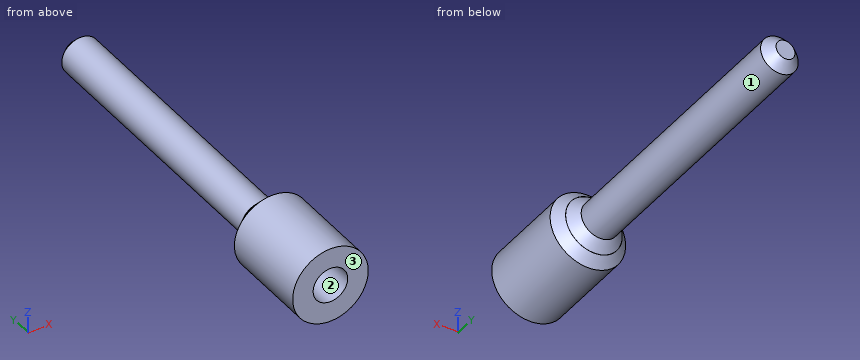
```python
from build123d import *

# Parameters (mm, degrees)
F0_R     = 101.843803
F0_R_2   = 46.640997
F1_DEPTH = 269.139469
F2_R     = 50.778729
F3_DEPTH = 801.080585
F4_SIZE  = 25.4


with BuildPart() as f1:
    # F0 (on Front) → F1 (new body)
    with BuildSketch(Plane.XZ):
        Circle(F0_R)
        Circle(F0_R_2, mode=Mode.SUBTRACT)
    extrude(amount=F1_DEPTH)

    # F2 (on Front) → F3 (join)
    with BuildSketch(Plane.XZ):
        Circle(F2_R)
    extrude(amount=-F3_DEPTH)

    # F4
    f4_edges = [f1.edges().sort_by_distance(p)[0] for p in [
        (50.778729, 400.540292, 0),
        (-50.778729, 0, 0),
        (-50.778729, 801.080585, 0),
        (-101.843803, 0, 0),
    ]]
    chamfer(f4_edges, length=F4_SIZE)


solid = f1.part
```
Design review of the part built by this model. Coordinates are the model's own, in mm. Face numbers are marked on the shaded views. Round coordinates to 2 decimals unless told otherwise and drop trailing zeros. Write each loop counter-clockwise with the first axis right and the second up, starting at its lowest first coordinate (ties: lowest second). Pieces come first, ordered by that corner, then holes. Notation, with made-up numbers: (33.5, 72.5) -> (69.5, 72.5) arc R32 ccw to (69.5, 103.5) -> close; hole circle Ø4 at (42.25, 67). An arc over 180 degrees is marked (long way). Write item = value, one per line. Start each with the question number.
1) Wall thickness on probe 1 along Z at (x, y) = (0, -107.5); probe 2 along Z at (x, y) = (-42, -128.5); probe 3 along Y at (x, z) = (-7, -65): over which ranges is each line inside the solid? List them lowest first. Write a range as from..to.
2) Take a section at A-A, the plane x = 0. State the section outline as (y, z) points, plus the area to 3 significant figures.
3) Take a section at C-C, the plane z = 0. State the section outline as (x, y) points.
4) Mouldability with a two-part tool opening along X and no side actions: class the marked faces 1, 2 and 3 as +X half, -X half, draft (parallel to the pull), parting line (faces both ways), or undercut.
5) Take a section at B-B, the plane y = -183.5. State the section outline as (x, z) points, plus the area to 3 significant figures.
6) Clearance check with flat-ended pins moving along their axes: pin 1 (5 mm diameter, centred on x = -18, y = 542.5, fed in from +Z); pin 2 (4 mm diameter, centred on x = -54, z = 76, fed in from +Y); pin 3 (3 mm diameter, centred on x = 77, y = -67, fed in from -Z). State where each tip first meets the part, or that it passes through.
7) Take a section at D-D, the plane y = 250. State the section outline as (x, z) points.
Results list:
q1.probe_1 = -101.84..-46.64, 46.64..101.84
q1.probe_2 = -92.78..-20.28, 20.28..92.78
q1.probe_3 = -269.14..10.8
q2.outline = (-269.14, -101.84) -> (-25.4, -101.84) -> (0, -76.44) -> (0, -76.18) -> (25.4, -50.78) -> (775.68, -50.78) -> (801.08, -25.38) -> (801.08, 25.38) -> (775.68, 50.78) -> (25.4, 50.78) -> (0, 76.18) -> (0, 76.44) -> (-25.4, 101.84) -> (-269.14, 101.84) -> (-269.14, 46.64) -> (0, 46.64) -> (0, -46.64) -> (-269.14, -46.64) -> close
q2.area = 110,000 mm²
q3.outline = (-101.84, -269.14) -> (-46.64, -269.14) -> (-46.64, 0) -> (46.64, 0) -> (46.64, -269.14) -> (101.84, -269.14) -> (101.84, -25.4) -> (76.44, 0) -> (76.18, 0) -> (50.78, 25.4) -> (50.78, 775.68) -> (25.38, 801.08) -> (-25.38, 801.08) -> (-50.78, 775.68) -> (-50.78, 25.4) -> (-76.18, 0) -> (-76.44, 0) -> (-101.84, -25.4) -> close
q4.face_1 = parting line
q4.face_2 = undercut
q4.face_3 = draft
q5.outline = circle Ø203.69 at (0, 0); hole circle Ø93.28 at (0, 0)
q5.area = 25,800 mm²
q6.pin_1 = 48.36
q6.pin_2 = -14.79
q6.pin_3 = -68.35
q7.outline = circle Ø101.56 at (0, 0)
